from build123d import *

# Parameters (mm, degrees)
F0_R          = 125
F0_R_2        = 25
F1_DEPTH      = 250
F3_DEPTH      = 100
F5_R          = 20
F6_DEPTH      = 40
F6_DEPTH_BACK = 10


with BuildPart() as f1:
    # F0 (on Front) → F1 (new body)
    with BuildSketch(Plane.XZ):
        Circle(F0_R)
        Circle(F0_R_2, mode=Mode.SUBTRACT)
    extrude(amount=F1_DEPTH)

    # F2 (on Front) → F3 (cut)
    with BuildSketch(Plane.XZ):
        with BuildLine():
            Line((-65, 20), (-83, 20))
            ThreePointArc((-83, 20), (-84.414214, 19.414214), (-85, 18))
            Line((-85, 18), (-85, 17))
            ThreePointArc((-85, 17), (-84.414214, 15.585786), (-83, 15))
            Line((-83, 15), (-81, 15))
            ThreePointArc((-81, 15), (-79.585786, 14.414214), (-79, 13))
            Line((-79, 13), (-79, -13))
            ThreePointArc((-79, -13), (-79.585786, -14.414214), (-81, -15))
            Line((-81, -15), (-83, -15))
            ThreePointArc((-83, -15), (-84.414214, -15.585786), (-85, -17))
            Line((-85, -17), (-85, -18))
            ThreePointArc((-85, -18), (-84.414214, -19.414214), (-83, -20))
            Line((-83, -20), (-65, -20))
            Line((-65, -20), (-65, 20))
        make_face()
    extrude(amount=F3_DEPTH, mode=Mode.SUBTRACT)

    # F5 (on offset) → F6 (join, two sides)
    with BuildSketch(Plane.YZ.offset(125)) as f6_sk:
        with Locations((-230, 0)):
            Circle(F5_R)
    extrude(amount=F6_DEPTH)
    extrude(f6_sk.sketch, amount=-F6_DEPTH_BACK)


solid = f1.part
Geometry: final body of the model. Coordinates: model frame, mm. A direction names the side the tool comes from. Give positions to 0.01 mm unless a question says otherwise; leave off trailing zeros. Write each loop counter-clockwise with the first axis right and the second up, starting at its lowest first coordinate (ties: lowest second). Pieces come first, ordered by that corner, then holes.
(1) First-contact query: P1, Ø2, axis at y = -25.5, z = -41, coming from the +X side; P2, Ø4, axis at x = -20.5, y = -91, coming from the -Z side; P3, Ø6, axis at x = -81, y = -160.5, coming from the -Z side. Flat tips, straight axial feed; report the tip coordinate or a pass-through.
(2) Access query for faces 5 (the flat face through (-2, 0, -26)), 6 (the flat face through (-74, -49, -20)). Directions: +Z, -Z, +X, -X, +Y, -Y. A direction counts if a zero-diameter tool reaches every point of the face in a straight line with its end or side. Return the directions, or none.
(3) Mould query, pull axis Z, two halves, no side actions, for faces 1 (the flat face through (165, -230, 0)), 2 (the cylindrical face through (-124.88, -123.25, 5.5)), 3 (the flat face through (-65, -49, 0)), 4 (the flat face through (-74, -49, 20)). Classes: released by +Z, released by -Z, zero draft, split by the parting line, or undercut.
(4) Cut plane B-B, the plane y = -80. Return loops of the section in (x, z).
(5) Ray query, line 1 (X direction, y = -77, z = -11.5); line 2 (Z direction, x = -106, y = -209.5); line 3 (Z direction, x = -43.5, y = -85). Return the intervals inside material, ascending.
(6) Cut plane C-C, the plane y = -230. Return loops of the section in (x, z), then the cut area to 3 significant figures.
(7) Cut plane D-D, the plane z = 79.5. Return loops of the section in (x, y), then the cut area to 3 significant figures.
(8) Cut plane A-A, the plane x = 0. Return loops of the section in (y, z).
Values follow:
1. P1: stops at x = 118.43
1. P2: stops at z = -123.62
1. P3: stops at z = -97.68
2. face 5: +Z, -Z, +X, -X, +Y
2. face 6: +Y
3. face 1: zero draft
3. face 2: split by the parting line
3. face 3: undercut
3. face 4: undercut
4. outline: circle Ø250 at (0, 0); hole (-85, -18) arc R2 ccw to (-83, -20) - (-65, -20) - (-65, 20) - (-83, 20) arc R2 ccw to (-85, 18) - (-85, 17) arc R2 ccw to (-83, 15) - (-81, 15) arc R2 cw to (-79, 13) - (-79, -13) arc R2 cw to (-81, -15) - (-83, -15) arc R2 ccw to (-85, -17) - close; hole circle Ø50 at (0, 0)
5. line 1: x = -124.47 to -79, -65 to -22.2, 22.2 to 124.47
5. line 2: z = -66.25 to 66.25
5. line 3: z = -117.19 to 117.19
6. outline: (123.39, -20) - (165, -20) - (165, 20) - (123.39, 20) arc R125 ccw (long way) to start; hole circle Ø50 at (0, 0)
6. area: 48,700 mm2
7. outline: (-96.46, -250) - (96.46, -250) - (96.46, 0) - (-96.46, 0) - close
7. area: 48,200 mm2
8. outline: (-250, -125) - (0, -125) - (0, -25) - (-250, -25) - close; (-250, 25) - (0, 25) - (0, 125) - (-250, 125) - close
